```python
from build123d import *

# Parameters (mm, degrees)
SKETCH_1_W          = 7.8
SKETCH_1_H          = 4
EXTRUDE_1_DEPTH     = 9
SKETCH_2_W          = 0.5
SKETCH_2_H          = 9
CUT_EXTRUDE_1_DEPTH = 1.8
FILLET_START        = -1
FILLET_1_DEPTH      = 11
FILLET_1_2_DEPTH    = 9
SHELL_1_T           = -0.5
SKETCH_3_W          = 4
SKETCH_3_H          = 1.5
EXTRUDE_2_DEPTH     = 7.5
CHAMFER_1_SIZE      = 1
CHAMFER_1_SIZE2     = 0.267949192
CHAMFER_2_SIZE      = 1
CHAMFER_2_SIZE2     = 0.267949192
SKETCH_4_W          = 1.5
SKETCH_4_H          = 0.896951392
EXTRUDE_3_DEPTH     = 0.2
SKETCH_5_W          = 1.5
SKETCH_5_H          = 0.2
EXTRUDE_4_DEPTH     = 1.5


with BuildPart() as part:
    # 草图1 → 拉伸1 (new body)
    with BuildSketch(Plane.XY):
        Rectangle(SKETCH_1_W, SKETCH_1_H)
    extrude(amount=EXTRUDE_1_DEPTH)

    # 草图2 → 切除-拉伸1 (cut)
    with BuildSketch(Plane.XZ.offset(2)):
        with Locations((-3.65, 4.5)):
            Rectangle(SKETCH_2_W, SKETCH_2_H)
        with Locations((3.65, 4.5)):
            Rectangle(SKETCH_2_W, SKETCH_2_H)
    extrude(amount=-CUT_EXTRUDE_1_DEPTH, mode=Mode.SUBTRACT)

    # 圆角1: read off the stored shape, not the designer's step
    # 圆角1 outline → 圆角1 (cut)
    with BuildSketch(Plane.XY.offset(FILLET_START)):
        with BuildLine():
            ThreePointArc((3.9, 0.05), (3.826776695, -0.126776695), (3.65, -0.2))
            Line((3.65, -0.2), (3.9, -0.2))
            Line((3.9, -0.2), (3.9, 0.05))
        make_face()
        with BuildLine():
            ThreePointArc((-3.65, -0.2), (-3.826776695, -0.126776695), (-3.9, 0.05))
            Line((-3.9, 0.05), (-3.9, -0.2))
            Line((-3.9, -0.2), (-3.65, -0.2))
        make_face()
    extrude(amount=FILLET_1_DEPTH, mode=Mode.SUBTRACT)

    # Fillet 1 2 outline → Fillet 1 2 (add)
    with BuildSketch(Plane.XY):
        with BuildLine():
            Line((3.4, -0.2), (3.4, -0.45))
            ThreePointArc((3.4, -0.45), (3.473223305, -0.273223305), (3.65, -0.2))
            Line((3.65, -0.2), (3.4, -0.2))
        make_face()
        with BuildLine():
            Line((-3.4, -0.2), (-3.65, -0.2))
            ThreePointArc((-3.65, -0.2), (-3.473223305, -0.273223305), (-3.4, -0.45))
            Line((-3.4, -0.45), (-3.4, -0.2))
        make_face()
    extrude(amount=FILLET_1_2_DEPTH)

    # 抽壳1
    shell_1_openings = [part.faces().sort_by_distance(p)[0] for p in [
        (0, 0.067245036, 9),
    ]]
    offset(amount=SHELL_1_T, openings=shell_1_openings, kind=Kind.INTERSECTION)

    # 草图3 → 拉伸2 (add)
    with BuildSketch(Plane.XY.offset(0.5)):
        with Locations((0, -0.25)):
            Rectangle(SKETCH_3_W, SKETCH_3_H)
    extrude(amount=EXTRUDE_2_DEPTH)

    # 倒角1
    chamfer_1_edges = [part.edges().sort_by_distance(p)[0] for p in [
        (-2, -1, 4.25),
    ]]
    chamfer_1_side = [part.faces().sort_by_distance(p)[0] for p in [
        (-2, -0.25, 4.25),
    ]]
    chamfer(chamfer_1_edges, length=CHAMFER_1_SIZE, length2=CHAMFER_1_SIZE2, reference=chamfer_1_side[0])

    # 倒角2
    chamfer_2_edges = [part.edges().sort_by_distance(p)[0] for p in [
        (2, -1, 4.25),
    ]]
    chamfer_2_side = [part.faces().sort_by_distance(p)[0] for p in [
        (2, -0.25, 4.25),
    ]]
    chamfer(chamfer_2_edges, length=CHAMFER_2_SIZE, length2=CHAMFER_2_SIZE2, reference=chamfer_2_side[0])

    # 草图4 → 拉伸3 (add)
    with BuildSketch(Plane(origin=(3.4, 0, 0), x_dir=(0, 0, -1), z_dir=(1, 0, 0))):
        with Locations((-6.05, -1.551524304)):
            Rectangle(SKETCH_4_W, SKETCH_4_H)
        with Locations((-0.75, -1.551524304)):
            Rectangle(SKETCH_4_W, SKETCH_4_H)
    extrude_3 = extrude(amount=EXTRUDE_3_DEPTH)

    # 镜向1: 拉伸3 across plane
    add(extrude_3.mirror(Plane(origin=(0, 0, 0), x_dir=(0, 0, 1), z_dir=(1, 0, 0))))

    # 草图5 → 拉伸4 (add)
    with BuildSketch(Plane(origin=(3.6, 0, 0), x_dir=(0, 0, -1), z_dir=(1, 0, 0))):
        with Locations((-6.05, -1.9)):
            Rectangle(SKETCH_5_W, SKETCH_5_H)
        with Locations((-0.75, -1.9)):
            Rectangle(SKETCH_5_W, SKETCH_5_H)
    extrude_4 = extrude(amount=EXTRUDE_4_DEPTH)

    # 镜向2: 拉伸4 across plane
    add(extrude_4.mirror(Plane(origin=(0, 0, 0), x_dir=(0, 0, 1), z_dir=(1, 0, 0))))


solid = part.part
```
Here's how the part is built. I have some questions about the finished solid (model axes, mm). A direction names the side the tool comes from. Coordinates: 2 decimals unless noted, no trailing zeros. Order: outer loops, then holes, each group sorted by start corner. A loop starts at its lowest first (then second) coordinate and runs counter-clockwise, first axis right, second up.
1) Imagine slicing it at A-A on z = 3.5. List the corners of the cut face in (x, y) for me.
2) Imagine slicing it at C-C on x = 2.25. List the corners of the cut face in (y, z) for me, and give its area (3 significant figures).
3) Will these pins go through, and if not, where does the flat tip stop? pin 1 (0.7 mm diameter, centred on x = 4.5, y = -1.5, fed in from +Z); pin 2 (1.2 mm diameter, centred on x = -0.5, y = 0, fed in from +Z); pin 3 (1.2 mm diameter, centred on y = -1, z = 6.5, fed in from -X).
4) Imagine slicing it at B-B on x = 4.5. List the corners of the cut face in (y, z) for me.
5) Imagine slicing it at D-D on y = 1.1. List the corners of the cut face in (x, z) for me, and give its area (3 significant figures).
6) I need wall thicknesses on line 1 (X direction, y = 0.3, z = 4.5); line 2 (Y direction, x = 1.5, z = 4.5); line 3 (Y direction, x = 2.5, z = 5.75). Which ranges of each line are inside material? Lowest first, please.
7) Which directions (+Z, -Z, +X, -X, +Y, -Y) give clear straight access to the entire face, cutting with the end or side of a thin tool? Please do faces 1 (the face through (-3.9, 1, 4)), 2 (the face through (0, 2, 4)), 3 (the face through (4, -1.8, 1)), 4 (the face through (1.864, -0.507, 4.198)).
8) We'd pull the mould along Z, two halves only. Please class faces 5 (the face through (4, -1.8, 6)), 6 (the face through (0, 0, 8)), 7 (the face through (3.4, -1, 4)): +Z half, -Z half, draft (parallel to the pull), parting line (faces both ways), or undercut.
Response values:
1. outline: (-3.9, 0.05) arc R0.25 ccw to (-3.65, -0.2) arc R0.25 cw to (-3.4, -0.45) - (-3.4, -2) - (3.4, -2) - (3.4, -0.45) arc R0.25 cw to (3.65, -0.2) arc R0.25 ccw to (3.9, 0.05) - (3.9, 2) - (-3.9, 2) - close; (-2, 0) - (-1.73, -1) - (1.73, -1) - (2, 0) - (2, 0.5) - (-2, 0.5) - close; hole (-3.4, 0.26) arc R0.75 cw to (-2.9, -0.45) - (-2.9, -1.5) - (2.9, -1.5) - (2.9, -0.45) arc R0.75 cw to (3.4, 0.26) - (3.4, 1.5) - (-3.4, 1.5) - close
2. outline: (-2, 0) - (2, 0) - (2, 9) - (1.5, 9) - (1.5, 0.5) - (-1.5, 0.5) - (-1.5, 9) - (-2, 9) - close
2. area: 10.5 mm2
3. pin 1: stops at z = 6.8
3. pin 2: stops at z = 8
3. pin 3: stops at x = -3.6
4. outline: (-2, 0) - (-1.8, 0) - (-1.8, 1.5) - (-2, 1.5) - close; (-2, 5.3) - (-1.8, 5.3) - (-1.8, 6.8) - (-2, 6.8) - close
5. outline: (-3.9, 0) - (3.9, 0) - (3.9, 9) - (3.4, 9) - (3.4, 0.5) - (-3.4, 0.5) - (-3.4, 9) - (-3.9, 9) - close
5. area: 12.4 mm2
6. line 1: x = -3.9 to -3.4, -2 to 2, 3.4 to 3.9
6. line 2: y = -2 to -1.5, -1 to 0.5, 1.5 to 2
6. line 3: y = -2 to -1.5, 1.5 to 2
7. face 1: +Z, -Z, -X, +Y
7. face 2: +Z, -Z, +X, -X, +Y
7. face 3: +Z, -Z, +X
7. face 4: +Z
8. face 5: draft
8. face 6: +Z half
8. face 7: undercut
